```python
from build123d import *

# Parameters (mm, degrees)
BOSS_EXTRUDE1_DEPTH = 4
FILLET1_R           = 10
CUT_EXTRUDE1_DEPTH  = 10


with BuildPart() as part:
    # Sketch1 → Boss-Extrude1 (new body)
    with BuildSketch(Plane(origin=(0, 0, 0), x_dir=(1, 0, 0), z_dir=(0, 1, 0))):
        with BuildLine():
            Line((-20, 11.278847861), (-20, -75))
            Line((-20, -75), (20, -75))
            Line((20, -75), (20, 11.278847861))
            ThreePointArc((20, 11.278847861), (34.67002501, 55.835487295), (72.941176471, 82.961539667))
            ThreePointArc((72.941176471, 82.961539667), (124.230373948, 108.248410071), (165, 148.346354961))
            Line((165, 148.346354961), (144.861111111, 163.159361217))
            ThreePointArc((144.861111111, 163.159361217), (89.963208148, 116.688216317), (20, 100))
            Line((20, 100), (-20, 100))
            ThreePointArc((-20, 100), (-89.963208148, 116.688216317), (-144.861111111, 163.159361217))
            Line((-144.861111111, 163.159361217), (-165, 148.346354961))
            ThreePointArc((-165, 148.346354961), (-124.230373948, 108.248410071), (-72.941176471, 82.961539667))
            ThreePointArc((-72.941176471, 82.961539667), (-34.67002501, 55.835487295), (-20, 11.278847861))
        make_face()
    extrude(amount=BOSS_EXTRUDE1_DEPTH)

    # Fillet1
    fillet1_edges = [part.edges().sort_by_distance(p)[0] for p in [
        (-165, 2, -148.346354961),
        (165, 2, -148.346354961),
    ]]
    fillet(fillet1_edges, radius=FILLET1_R)

    # Sketch2 → Cut-Extrude1 (cut)
    with BuildSketch(Plane(origin=(0, 4, 0), x_dir=(1, 0, 0), z_dir=(0, 1, 0))):
        with BuildLine():
            Line((3.2, 40), (3.2, -5))
            ThreePointArc((3.2, -5), (0, -8.2), (-3.2, -5))
            Line((-3.2, -5), (-3.2, 40))
            ThreePointArc((-3.2, 40), (0, 43.2), (3.2, 40))
        make_face()
        with BuildLine():
            Line((3.2, -20), (3.2, -65))
            ThreePointArc((3.2, -65), (0, -68.2), (-3.2, -65))
            Line((-3.2, -65), (-3.2, -20))
            ThreePointArc((-3.2, -20), (0, -16.8), (3.2, -20))
        make_face()
    extrude(amount=-CUT_EXTRUDE1_DEPTH, mode=Mode.SUBTRACT)


solid = part.part
```
Can you work these out from the model? Positions are in its coordinate system, mm. A direction names the side the tool comes from. Give positions to 0.01 mm unless a question says otherwise; leave off trailing zeros. Order: outer loops, then holes, each group sorted by start corner. A loop starts at its lowest first (then second) coordinate and runs counter-clockwise, first axis right, second up. Notation, with made-up numbers: M 50,50.25 L 67,50.25 A26 cw 67,81.25 Z; hole C 22.5,-14.5 d10. An arc over 180 degrees is marked long. Write item = value, one per line. Start each with the question number.
Q1. We'd pull the mould along X, two halves only. Please class faces 3 (the cylindrical face through (90.87, 1.97, -117.15)), 4 (the cylindrical face through (119.26, 1.97, -104.84)), 5 (the cylindrical face through (-35.07, 1.97, -56.37)): pulls with the +X half, pulls with the -X half, needs draft (parallel to the pull), parting line crosses it, or undercut.
Q2. Will these pins go through, and if not, where does the flat tip stop? pin 1 Ø1.2 at (y, z) = (2, 36) entering from -X; pin 2 Ø1.2 at (y, z) = (2.5, -25) entering from +X; pin 3 Ø2 at (y, z) = (1.5, 50.5) entering from +X.
Q3. I need wall thicknesses on probe 1 along X at (y, z) = (2.5, 37); probe 2 along X at (y, z) = (0.65, -28); probe 3 along X at (y, z) = (1.35, 8.5). Which ranges of each line are inside material? Lowest first, please. Write a range as [from, to].
Q4. For faces 1 (the flat face through (-150.701, 1.972, -158.864)), 2 (the cylindrical face through (-89.05, 1.97, -116.23)), which set-ups out of +Z, -Z, +X, -X, +Y, -Y let a thin tool reach every point of the face, with its end or its side?
Q5. Suppose I cut it at B-B (z = -131.5). Write out the boundary of the cut face in (x, y).
Q6. Suppose I cut it at C-C (z = 13). Write out the boundary of the cut face in (x, y).
Q7. Suppose I cut it at D-D (x = 59). Write out the boundary of the cut face in (y, z), plus the area to 3 significant figures.
Q8. Suppose I cut it at A-A (y = 0.7). Write out the boundary of the cut face in (x, z), plus the area to 3 significant figures.
Check result:
q1.face_3 = undercut
q1.face_4 = pulls with the +X half
q1.face_5 = pulls with the -X half
q2.pin_1 = -20
q2.pin_2 = 21.38
q2.pin_3 = 20
q3.probe_1 = [-20, -3.2], [3.2, 20]
q3.probe_2 = [-21.89, -3.2], [3.2, 21.89]
q3.probe_3 = [-20, 20]
q4.face_1 = -Z, -X, +Y, -Y
q4.face_2 = -Z, +Y, -Y
q5.outline = M -150.95,0 L -113.66,0 L -113.66,4 L -150.95,4 Z; M 113.66,0 L 150.95,0 L 150.95,4 L 113.66,4 Z
q6.outline = M -20,0 L 20,0 L 20,4 L -20,4 Z
q7.outline = M 0,-104.99 L 4,-104.99 L 4,-77.07 L 0,-77.07 Z
q7.area = 112 mm2
q8.outline = M -158.48,-140 A10 ccw -156.71,-154.45 L -144.86,-163.16 A155 cw -20,-100 L 20,-100 A155 cw 144.86,-163.16 L 156.71,-154.45 A10 ccw 158.48,-140 A180 ccw 72.94,-82.96 A75 cw 20,-11.28 L 20,75 L -20,75 L -20,-11.28 A75 cw -72.94,-82.96 A180 ccw Z; hole M -3.2,-40 A3.2 ccw 3.2,-40 L 3.2,5 A3.2 ccw -3.2,5 Z; hole M -3.2,20 A3.2 ccw 3.2,20 L 3.2,65 A3.2 ccw -3.2,65 Z
q8.area = 15,600 mm2
